Geometry check sheet. Reference: the model listing, model coordinates, mm. Face numbers are marked on the shaded views. A direction names the side the tool comes from. Coordinates: 2 decimals unless noted, no trailing zeros. Loops run counter-clockwise (first coordinate to the right, second up) from the corner with the lowest first, then second, coordinate; pieces in that order, holes last. Notation, with made-up numbers: (0, 34.25) -> (25, 34.25) arc R21 cw to (25, 53.25) -> close; hole circle Ø6 at (-31, -8). An arc over 180 degrees is marked (long way). Answer as a JSON object with one key per item and string values.
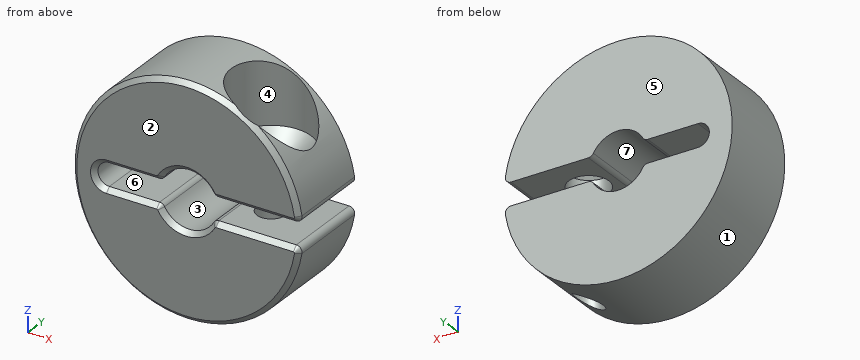
from build123d import *

# Parameters (mm, degrees)
SKETCH1_R               = 10
SKETCH1_R_2             = 2.5
BOSS_EXTRUDE1_DEPTH     = 3.75
CUT_EXTRUDE1_DEPTH      = 17.007810594
CUT_EXTRUDE2_DEPTH      = 16.331748106
CUT_EXTRUDE2_DEPTH_BACK = 16.331748106
SKETCH3_R               = 1.25
SKETCH4_R               = 1.75
CUT_EXTRUDE3_DEPTH      = 16.331748268
CUT_EXTRUDE4_START      = 6
SKETCH5_R               = 3.5
CUT_EXTRUDE4_DEPTH      = 8
CHAMFER1_SIZE           = 2.5
FILLET1_R               = 0.5
CHAMFER2_SIZE           = 0.4


with BuildPart() as part:
    # Sketch1 → Boss-Extrude1 (new, symmetric)
    with BuildSketch(Plane(origin=(0, 0, 0), x_dir=(1, 0, 0), z_dir=(0, 1, 0))):
        with Locations(Location((0, 0, 0), (0, 0, 270))):
            Circle(SKETCH1_R)
        with Locations(Location((0, 0, 0), (0, 0, 270))):
            Circle(SKETCH1_R_2, mode=Mode.SUBTRACT)
    extrude(amount=BOSS_EXTRUDE1_DEPTH, both=True)

    # Sketch2 → Cut-Extrude1 (cut, through all)
    with BuildSketch(Plane(origin=(0, 3.75, 0), x_dir=(1, 0, 0), z_dir=(0, 1, 0))):
        with BuildLine():
            Line((10, -1), (-7, -1))
            ThreePointArc((-7, -1), (-8, 0), (-7, 1))
            Line((-7, 1), (10, 1))
            ThreePointArc((10, 1), (11, 0), (10, -1))
        make_face()
    extrude(amount=-CUT_EXTRUDE1_DEPTH, mode=Mode.SUBTRACT)

    # Sketch3 → Cut-Extrude2 (cut, two sides: drawn at the far end of the back side and taken through both)
    with BuildSketch(Plane.XY.offset(-1).offset(-CUT_EXTRUDE2_DEPTH_BACK)):
        with Locations((5, 0)):
            Circle(SKETCH3_R)
    extrude(amount=CUT_EXTRUDE2_DEPTH + CUT_EXTRUDE2_DEPTH_BACK, mode=Mode.SUBTRACT)

    # Sketch4 → Cut-Extrude3 (cut, through all)
    with BuildSketch(Plane.XY.offset(-1)):
        with Locations(Location((5, 0, 0), (0, 0, 180))):
            Circle(SKETCH4_R)
    extrude(amount=CUT_EXTRUDE3_DEPTH, mode=Mode.SUBTRACT)

    # Sketch5 → Cut-Extrude4 (cut)
    with BuildSketch(Plane.XY.offset(-1).offset(CUT_EXTRUDE4_START)):
        with Locations(Location((5, 0, 0), (0, 0, 180))):
            Circle(SKETCH5_R)
    extrude(amount=CUT_EXTRUDE4_DEPTH, mode=Mode.SUBTRACT)

    # Chamfer1
    # the kernel refuses this chamfer: 2.5 mm, written as the material it takes off along each edge
    with BuildSketch(Plane(origin=(5, 0, 5), x_dir=(-1, 0, 0), z_dir=(0, -1, 0))) as chamfer1_piece_1_section:
        Polygon((1.75, CHAMFER1_SIZE), (1.75 + CHAMFER1_SIZE, 0), (1.75, 0), align=None)
    chamfer1_piece_1 = revolve(axis=Axis((5, 0, 5), (0, 0, -1)), mode=Mode.PRIVATE)
    chamfer1_piece_1 = chamfer1_piece_1 & Plane(origin=(5, 0, 3.399981632), x_dir=(-1, 0, 0), z_dir=(0, 0, -1)) * Cylinder(3.5, 17, mode=Mode.PRIVATE)
    add(chamfer1_piece_1, mode=Mode.SUBTRACT)

    # Fillet1
    fillet1_edges = [part.edges().sort_by_distance(p)[0] for p in [
        (-2.291287847, 0, -1),
        (2.291287847, 0, -1),
        (2.291287847, 0, 1),
        (-2.291287847, 0, 1),
        (9.949874371, 0, 1),
        (9.949874371, 0, -1),
    ]]
    fillet(fillet1_edges, radius=FILLET1_R)

    # Chamfer2
    # the kernel refuses this chamfer: 0.4 mm, written as the material it takes off along each edge
    with BuildSketch(Plane(origin=(9.38083152, -3.75, 1.5), x_dir=(0.9874559494365127, 0, 0.15789473684209784), z_dir=(-0.15789473684209784, 0, 0.9874559494365127))) as chamfer2_piece_1:
        Polygon((0.5, CHAMFER2_SIZE), (0.5 - CHAMFER2_SIZE, 0), (0.5, 0), align=None)
    revolve(axis=Axis((9.38083152, -3.75, 1.5), (0, 1, 0)), revolution_arc=99.084720287, mode=Mode.SUBTRACT)
    with BuildSketch(Plane(origin=(0, -3.75, 0), x_dir=(0.9874559494365116, 0, -0.15789473684210514), z_dir=(0.15789473684210514, 0, 0.9874559494365116))) as chamfer2_piece_2:
        Polygon((10, CHAMFER2_SIZE), (10 - CHAMFER2_SIZE, 0), (10, 0), align=None)
    revolve(axis=Axis((0, -3.75, 0), (0, 1, 0)), revolution_arc=341.830559425, mode=Mode.SUBTRACT)
    with BuildSketch(Plane(origin=(9.38083152, -3.75, 1), x_dir=(0, -0.027495876610586285, 0.9996219169112968), z_dir=(-1, 0, 0)), Plane(origin=(2.598076211, -3.75, -1), x_dir=(0, -0.027495876610586285, -0.9996219169112968), z_dir=(1, 0, 0))) as chamfer2_piece_3:
        Polygon((CHAMFER2_SIZE * 0.999621916911, CHAMFER2_SIZE * 0.0274958766106), (-CHAMFER2_SIZE * 0.0274958766106, CHAMFER2_SIZE * 0.999621916911), (0, 0), align=None)
    extrude(amount=6.782755308, mode=Mode.SUBTRACT)
    with BuildSketch(Plane(origin=(9.38083152, -3.75, -1.5), x_dir=(0.9874559494365118, 0, -0.1578947368421039), z_dir=(-0.1578947368421039, 0, -0.9874559494365118))) as chamfer2_piece_4:
        Polygon((0.5, -CHAMFER2_SIZE), (0.5 - CHAMFER2_SIZE, 0), (0.5, 0), align=None)
    revolve(axis=Axis((9.38083152, -3.75, -1.5), (0, -1, 0)), revolution_arc=99.084720287, mode=Mode.SUBTRACT)
    with BuildSketch(Plane(origin=(2.598076211, -3.75, 1.5), x_dir=(-0.8660254037844399, 0, -0.49999999999999767), z_dir=(-0.49999999999999767, 0, 0.8660254037844399))) as chamfer2_piece_5:
        Polygon((0.5 - CHAMFER2_SIZE, 0), (0.5, -CHAMFER2_SIZE), (0.5, 0), align=None)
    revolve(axis=Axis((2.598076211, -3.75, 1.5), (0, -1, 0)), revolution_arc=60, mode=Mode.SUBTRACT)
    with BuildSketch(Plane(origin=(0, -3.75, 0), x_dir=(-0.8660254037844383, 0, 0.5000000000000007), z_dir=(-0.5000000000000007, 0, -0.8660254037844383))) as chamfer2_piece_6:
        Polygon((2.5 + CHAMFER2_SIZE, 0), (2.5, CHAMFER2_SIZE), (2.5, 0), align=None)
    revolve(axis=Axis((0, -3.75, 0), (0, 1, 0)), revolution_arc=120, mode=Mode.SUBTRACT)
    with BuildSketch(Plane(origin=(2.598076211, -3.75, -1.5), x_dir=(-0.866025403784439, 0, 0.49999999999999944), z_dir=(-0.49999999999999944, 0, -0.866025403784439))) as chamfer2_piece_7:
        Polygon((0.5 - CHAMFER2_SIZE, 0), (0.5, CHAMFER2_SIZE), (0.5, 0), align=None)
    revolve(axis=Axis((2.598076211, -3.75, -1.5), (0, 1, 0)), revolution_arc=60, mode=Mode.SUBTRACT)
    with BuildSketch(Plane(origin=(-2.598076211, -3.75, 1.5), x_dir=(0, 0, -1), z_dir=(-1, 0, 0))) as chamfer2_piece_8:
        Polygon((0.5 - CHAMFER2_SIZE, 0), (0.5, -CHAMFER2_SIZE), (0.5, 0), align=None)
    revolve(axis=Axis((-2.598076211, -3.75, 1.5), (0, -1, 0)), revolution_arc=60, mode=Mode.SUBTRACT)
    with BuildSketch(Plane(origin=(0, -3.75, 0), x_dir=(0.8660254037844389, 0, -0.49999999999999967), z_dir=(0.49999999999999967, 0, 0.8660254037844389))) as chamfer2_piece_9:
        Polygon((2.5 + CHAMFER2_SIZE, 0), (2.5, CHAMFER2_SIZE), (2.5, 0), align=None)
    revolve(axis=Axis((0, -3.75, 0), (0, 1, 0)), revolution_arc=120, mode=Mode.SUBTRACT)
    with BuildSketch(Plane(origin=(-2.598076211, -3.75, 1), x_dir=(0, -0.027495876610586285, 0.9996219169112968), z_dir=(-1, 0, 0)), Plane(origin=(-7, -3.75, -1), x_dir=(0, -0.027495876610586275, -0.9996219169112966), z_dir=(1, 0, 0))) as chamfer2_piece_10:
        Polygon((CHAMFER2_SIZE * 0.999621916911, CHAMFER2_SIZE * 0.0274958766106), (-CHAMFER2_SIZE * 0.0274958766106, CHAMFER2_SIZE * 0.999621916911), (0, 0), align=None)
    extrude(amount=4.401923789, mode=Mode.SUBTRACT)
    with BuildSketch(Plane(origin=(-2.598076211, -3.75, -1.5), x_dir=(0.8660254037844403, 0, 0.4999999999999974), z_dir=(0.4999999999999974, 0, -0.8660254037844403))) as chamfer2_piece_11:
        Polygon((0.5 - CHAMFER2_SIZE, 0), (0.5, -CHAMFER2_SIZE), (0.5, 0), align=None)
    revolve(axis=Axis((-2.598076211, -3.75, -1.5), (0, -1, 0)), revolution_arc=60, mode=Mode.SUBTRACT)
    with BuildSketch(Plane(origin=(-7, -3.75, 0), x_dir=(0, 0, -1), z_dir=(1, 0, 0))) as chamfer2_piece_12:
        Polygon((1 + CHAMFER2_SIZE, 0), (1, CHAMFER2_SIZE), (1, 0), align=None)
    revolve(axis=Axis((-7, -3.75, 0), (0, 1, 0)), revolution_arc=180, mode=Mode.SUBTRACT)


solid = part.part
1. Section check C-C, the plane y = 0. Record the boundary of the cut face in (x, z), then the cut area to 3 significant figures.
Evaluation:
{"outline": "(-7, -1) arc R1 cw to (-7, 1) -> (-2.6, 1) arc R0.5 ccw to (-2.17, 1.25) arc R2.5 cw to (2.17, 1.25) arc R0.5 ccw to (2.6, 1) -> (3.25, 1) -> (3.25, 2.5) -> (1.5, 4.25) -> (1.5, 9.89) arc R10 ccw (long way) to (3.75, -9.27) -> (3.75, -1) -> (2.6, -1) arc R0.5 ccw to (2.17, -1.25) arc R2.5 cw to (-2.17, -1.25) arc R0.5 ccw to (-2.6, -1) -> close; (6.25, -7.81) arc R10 ccw to (9.87, -1.58) arc R0.5 ccw to (9.38, -1) -> (6.25, -1) -> close; (6.75, 1) -> (9.38, 1) arc R0.5 ccw to (9.87, 1.58) arc R10 ccw to (8.5, 5.27) -> (8.5, 4.25) -> (6.75, 2.5) -> close", "area": "207 mm^2"}
2. Section check D-D, the plane x = 5. State how many separate pieces and enclosed holes the cut face has, then the cut area to 3 significant figures.
Evaluation:
{"separate pieces": "4", "enclosed holes": "0", "area": "50.1 mm^2"}
3. Thickness scan on probe 1 along Y at (x, z) = (5, 2.05); probe 2 along Y at (x, z) = (5, -3); probe 3 along Z at (x, y) = (-6.75, 2). Record the ranges inside material, lowest first. Write a range as from..to.
Evaluation:
{"probe 1": "y = -3.75..-1.75, 1.75..3.75", "probe 2": "y = -3.75..-1.25, 1.25..3.75", "probe 3": "z = -7.38..-1, 1..7.38"}
4. Section check B-B, the plane z = 0. Record the boundary of the cut face in (x, y).
Evaluation:
{"outline": "(-10, -3.35) -> (-9.6, -3.75) -> (-8.4, -3.75) -> (-8, -3.35) -> (-8, 3.75) -> (-10, 3.75) -> close"}
5. Section check A-A, the plane x = 0. Record the boundary of the cut face in (y, z).
Evaluation:
{"outline": "(-3.75, -9.6) -> (-3.35, -10) -> (3.75, -10) -> (3.75, -2.5) -> (-3.35, -2.5) -> (-3.75, -2.9) -> close; (-3.75, 2.9) -> (-3.35, 2.5) -> (3.75, 2.5) -> (3.75, 10) -> (-3.35, 10) -> (-3.75, 9.6) -> close"}
6. Mould release check, pull along X, two halves, no side actions. Record for the marked faces 1, 2 and 3: released by +X, released by -X, zero draft, split by the parting line, or undercut.
Evaluation:
{"face 1": "split by the parting line", "face 2": "zero draft", "face 3": "undercut"}
7. Tool access check on the marked faces 4, 5, 6 and 7. Record the directions out of +Z, -Z, +X, -X, +Y, -Y that give a thin tool (end or side, any length) a straight path to the whole face; none if there is none.
Evaluation:
{"face 4": "+Z", "face 5": "+Z, -Z, +X, -X, +Y", "face 6": "+X, +Y, -Y", "face 7": "+Y, -Y"}
8. Depth check by flat-ended pin: P1, Ø1, axis at y = 2, z = 4.5, coming from the +X side; P2, Ø4, axis at x = 5, y = 0, coming from the +Z side; P3, Ø1.3, axis at x = -4, y = 1, coming from the +Z side. Enter the tip coordinate at first touch or a pass-through.
Evaluation:
{"P1": "stops at x = 9.17", "P2": "stops at z = 2.75", "P3": "stops at z = 9.42"}
